CAD build for the part. Positions are in the model's coordinates, mm. Face numbers are marked on the shaded views. Coordinates: 2 decimals unless noted, no trailing zeros. Order: outer loops, then holes, each group sorted by start corner. A loop starts at its lowest first (then second) coordinate and runs counter-clockwise, first axis right, second up. Notation, with made-up numbers: (82, -34.75) - (103, -34.75) arc R14 ccw to (103, -20.75) - close; hole circle Ø8 at (53, 61.5). An arc over 180 degrees is marked (long way). Write each question's results on one line, items separated by ' | '. Start each with the question number.
Q1. Band-saw the part on B-B, the plane z = 0. Write the cut outline in (x, y).
Q2. Band-saw the part on C-C, the plane y = 3.75. Count the separate pieces of the cut face and the enclosed holes in it, then the cut area to 3 significant figures.
Q3. Band-saw the part on D-D, the plane x = 14.5. Write the cut outline in (y, z), then the cut area to 3 significant figures.
Q4. Wall check: probe 1 along X at (y, z) = (3.6, 12.7); probe 2 along X at (y, z) = (1.95, 12.7); probe 3 along X at (y, z) = (3, 27). Give the ranges that are in metal, low to high.
Q5. Pin check, flat tips, straight feed: P1, Ø2.5, axis at x = 22, z = 12.7, coming from the -Y side; P2, Ø2, axis at y = 4, z = 25, coming from the -X side; P3, Ø6.5, axis at x = -1, z = -25.5, coming from the +Y side; P4, Ø5, axis at x = -22, z = 12.7, coming from the +Y side. Stop position of each tip, or through.
Q6. Pull direction Z, two halves, no side cores. Call the marked faces 1, 2 and 3: released by +Z, released by -Z, zero draft, split by the parting line, or undercut.
Q7. Band-saw the part on A-A, the plane x = 0. Write the cut outline in (y, z), then the cut area to 3 significant figures.
Autodesk Inventor part; units mm, degrees
ref_plane "YZ Plane" through (0, 0, 0) normal (1, 0, 0) x (0, 1, 0)
ref_plane "XZ Plane" through (0, 0, 0) normal (0, 1, 0) x (-1, 0, 0)
ref_plane "XY Plane" through (0, 0, 0) normal (0, 0, 1) x (1, 0, 0)
sketch "Sketch1" plane through (0, 0, 0) normal (0, 1, 0) x (-1, 0, 0)
  circle A0 centre (0, 0) radius 38.1
  circle A1 centre (0, 0) radius 19.05
  circle A2 centre (0, 0) radius 25.4 construction
  dimension "d0" = 50.8
  dimension "d1" = 6.35
  dimension "d5" = 76.2
extrude "Extrusion1" add sketch "Sketch1" along normal blind 5.08
sketch "Sketch2" plane through (0, 5.08, 0) normal (0, 1, 0) x (1, 0, 0)
  circle A0 centre (0, 0) radius 19.05
  point P0 (0, 25.4)
  dimension "d6" = 25.4
hole "Hole1" at (0, 5.08, -25.4) direction (0, -1, 0) diameter 3.048 end through all counterbore diameter 6.096 counterbore depth 2.54
pattern_circular "Circular Pattern1" count 3 over 360 about axis through (0, 0, 0) along (0, 1, 0) of "Hole1"
sketch "Sketch4" plane through (0, 5.08, 0) normal (0, 1, 0) x (1, 0, 0)
  circle A0 centre (0, 0) radius 19.05
  circle A1 centre (24.7446, 22.7186) radius 1.524
  circle A2 centre (-23.5154, 23.9886) radius 1.524
  circle A3 centre (-18.4354, -28.0814) radius 1.524
  circle A4 centre (9.5046, -28.0814) radius 1.524
  dimension "d17" = 3.048
  dimension "d18" = 27.94
  dimension "d19" = 15.24
  dimension "d20" = 5.08
  dimension "d21" = 50.8
  dimension "d22" = 1.27
  dimension "d23" = 33.5921
  dimension "d24" = 33.5921
  dimension "d25" = 33.5921
extrude "Extrusion2" cut sketch "Sketch4" against normal through all contours A1 | A2 | A3 | A4
sketch "Sketch5" plane through (0, 5.08, 0) normal (0, 1, 0) x (1, 0, 0)
  circle A0 centre (-18.4354, -28.0814) radius 1.524
  circle A1 centre (24.7446, 22.7186) radius 1.524
  circle A2 centre (-23.5154, 23.9886) radius 1.524
  circle A3 centre (9.5046, -28.0814) radius 1.524
  circle A4 centre (-23.5154, 23.9886) radius 2.8575
  circle A5 centre (24.7446, 22.7186) radius 2.8575
  circle A6 centre (9.5046, -28.0814) radius 2.8575
  circle A7 centre (-18.4354, -28.0814) radius 2.8575
  dimension "d28" = 5.715
extrude "Extrusion3" add sketch "Sketch5" along normal blind 2.54
equation "\"d23\" = d25"
equation "\"d24\" = d25"
properties part number "Arduino Mount"
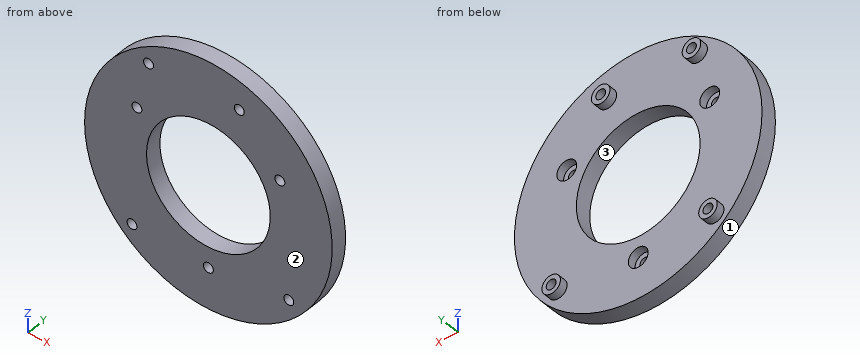
Results below:
1) outline: (-38.1, 0) - (-19.05, 0) - (-19.05, 5.08) - (-38.1, 5.08) - close; (19.05, 0) - (38.1, 0) - (38.1, 5.08) - (19.05, 5.08) - close
2) separate pieces: 1 | enclosed holes: 8 | area: 3,300 mm²
3) outline: (0, -35.23) - (5.08, -35.23) - (5.08, -12.36) - (0, -12.36) - close; (0, 12.36) - (5.08, 12.36) - (5.08, 35.23) - (0, 35.23) - close | area: 232 mm²
4) probe 1: x = -35.92 to -25.05, -18.95 to -14.2, 14.2 to 18.95, 25.05 to 35.92 | probe 2: x = -35.92 to -23.52, -20.47 to -14.2, 14.2 to 20.47, 23.52 to 35.92 | probe 3: x = -26.88 to -19.51, -17.36 to 8.43, 10.58 to 26.88
5) P1: passes through | P2: stops at x = -29.59 | P3: stops at y = 5.08 | P4: stops at y = 2.54
6) face 1: split by the parting line | face 2: zero draft | face 3: undercut
7) outline: (0, -38.1) - (5.08, -38.1) - (5.08, -28.45) - (2.54, -28.45) - (2.54, -26.92) - (0, -26.92) - close; (0, -23.88) - (2.54, -23.88) - (2.54, -22.35) - (5.08, -22.35) - (5.08, -19.05) - (0, -19.05) - close; (0, 19.05) - (5.08, 19.05) - (5.08, 38.1) - (0, 38.1) - close | area: 170 mm²
